```python
from build123d import *

# Parameters (mm, degrees)
F0_W      = 50
F0_H      = 40
F1_DEPTH  = 25
F2_W      = 40
F2_H      = 33
F3_DEPTH  = 25.001
F4_W      = 7
F4_H      = 25
F5_DEPTH  = 3
F6_R      = 1.25
F7_DEPTH  = 50.001
F8_W      = 25
F8_H      = 7
F9_DEPTH  = 5
F10_R     = 1.25
F11_DEPTH = 2
F12_R     = 3


with BuildPart() as f1:
    # F0 (on Front) → F1 (new body)
    with BuildSketch(Plane.XZ):
        with Locations((4.001731, 5.162706)):
            Rectangle(F0_W, F0_H)
    extrude(amount=F1_DEPTH)

    # F2 (on face) → F3 (cut, through all)
    with BuildSketch(Plane.XZ.offset(25)):
        with Locations((4.001731, 1.662706)):
            Rectangle(F2_W, F2_H)
    extrude(amount=-F3_DEPTH, mode=Mode.SUBTRACT)

    # F4 (on face) → F5 (cut)
    with BuildSketch(Plane.YZ.offset(-15.998269)):
        with Locations((-12.5, 1.662706)):
            Rectangle(F4_W, F4_H)
    extrude(amount=-F5_DEPTH, mode=Mode.SUBTRACT)

    # F6 (on face) → F7 (cut, through all)
    with BuildSketch(Plane(origin=(-20.998269, 0, 0), x_dir=(0, -1, 0), z_dir=(-1, 0, 0))):
        with Locations((12.5, -7.587294)):
            Circle(F6_R)
    extrude(amount=-F7_DEPTH, mode=Mode.SUBTRACT)

    # F8 (on face) → F9 (cut)
    with BuildSketch(Plane.XY.offset(25.162706)):
        with Locations((4.001731, -12.5)):
            Rectangle(F8_W, F8_H)
    extrude(amount=-F9_DEPTH, mode=Mode.SUBTRACT)

    # F10 (on face) → F11 (cut)
    with BuildSketch(Plane.XY.offset(20.162706)):
        with Locations((13.251731, -12.5)):
            Circle(F10_R)
    extrude(amount=-F11_DEPTH, mode=Mode.SUBTRACT)

    # F12
    f12_edges = [f1.edges().sort_by_distance(p)[0] for p in [
        (29.001731, -12.5, 25.162706),
        (-20.998269, -12.5, 25.162706),
        (4.001731, 0, 25.162706),
        (4.001731, -25, 25.162706),
        (29.001731, -25, 5.162706),
        (29.001731, 0, 5.162706),
        (-20.998269, -25, 5.162706),
        (-20.998269, 0, 5.162706),
        (-20.998269, -12.5, -14.837294),
        (29.001731, -12.5, -14.837294),
        (26.501731, -25, -14.837294),
        (-18.498269, -25, -14.837294),
        (26.501731, 0, -14.837294),
        (-18.498269, 0, -14.837294),
        (4.001731, -25, 18.162706),
        (4.001731, 0, 18.162706),
    ]]
    fillet(f12_edges, radius=F12_R)


solid = f1.part
```
Build history of the part. All positions in model axes, mm. A direction names the side the tool comes from. Give positions to 0.01 mm unless a question says otherwise; leave off trailing zeros. Loops run counter-clockwise (first coordinate to the right, second up) from the corner with the lowest first, then second, coordinate; pieces in that order, holes last.
1) Band-saw the part on D-D on x = -13. List the corners of the cut face in (y, z).
Values follow:
outline: (-25, 21.16) arc R3 ccw to (-22, 18.16) - (-3, 18.16) arc R3 ccw to (0, 21.16) - (0, 22.16) arc R3 ccw to (-3, 25.16) - (-22, 25.16) arc R3 ccw to (-25, 22.16) - close
2) 3-axis set-ups, long thin cutter, end or side, ignore diameter. For faces 1 (the face through (26.47, -11.58, -6.74)), 2 (the face through (-17, -9, 1)): which of +Z, -Z, +X, -X, +Y, -Y reach the whole face in a straight line?
Values follow:
face 1: +X, -X
face 2: none
3) Two-plate mould, pull along X, no slides. Class faces 3 (the face through (28.146, -12.633, -13.935)), 4 (the face through (-17, -13, -10.837)), 5 (the face through (4.31, -0.855, 24.261)), 6 (the face through (4, -12, 20.163)): released by +X, released by -X, zero draft, split by the parting line, or undercut.
Values follow:
face 3: released by +X
face 4: undercut
face 5: zero draft
face 6: undercut
4) Band-saw the part on A-A on y = -12.5. State how many separate pieces and enclosed holes the cut face has, then the cut area to 3 significant figures.
Values follow:
separate pieces: 4
enclosed holes: 0
area: 450 mm2
5) Band-saw the part on C-C on y = -6.5. List the corners of the cut face in (x, z), then the cut area to 3 significant figures.
Values follow:
outline: (-21, -11.84) arc R3 ccw to (-18, -14.84) - (-16, -14.84) - (-16, 18.16) - (24, 18.16) - (24, -14.84) - (26, -14.84) arc R3 ccw to (29, -11.84) - (29, 22.16) arc R3 ccw to (26, 25.16) - (-18, 25.16) arc R3 ccw to (-21, 22.16) - close
area: 672 mm2
6) Probe line 1 along X through (y, z) = (-14.75, -1.5); line 2 along X through (y, z) = (-8.5, 6); line 3 along Y through (x, z) = (12, 22). List the from-to ranges inside material, lowest first.
Values follow:
line 1: x = -21 to -19, 24 to 29
line 2: x = -21 to -16, 24 to 29
line 3: y = -25 to -16, -9 to 0
7) Band-saw the part on B-B on z = 5.5. List the corners of the cut face in (x, y), then the cut area to 3 significant figures.
Values follow:
outline: (-21, -22) arc R3 ccw to (-18, -25) - (-16, -25) - (-16, -16) - (-19, -16) - (-19, -9) - (-16, -9) - (-16, 0) - (-18, 0) arc R3 ccw to (-21, -3) - close; (24, -25) - (26, -25) arc R3 ccw to (29, -22) - (29, -3) arc R3 ccw to (26, 0) - (24, 0) - close
area: 221 mm2
8) Drop flat-ended pins along their axis: P1, Ø9.5, axis at x = -1, y = -13, coming from the -Z side; P2, Ø3, axis at y = -12.5, z = -7.59, coming from the -X side; P3, Ø1, axis at x = -13.5, z = 19, coming from the -Y side. Give the stop position or say it passes through.
Values follow:
P1: stops at z = 18.16
P2: stops at x = -21
P3: stops at y = -24.5
